Geometry check sheet. Reference: the model listing, model coordinates, mm. Face numbers are marked on the shaded views. A direction names the side the tool comes from. Coordinates: 2 decimals unless noted, no trailing zeros. Loops run counter-clockwise (first coordinate to the right, second up) from the corner with the lowest first, then second, coordinate; pieces in that order, holes last.
from build123d import *

# Parameters (mm, degrees)
BOSS_EXTRUDE1_DEPTH = 167.4876
FILLET1_R           = 4.7625
SHELL2_T            = -3.175
SKETCH2_R           = 25.4
CUT_EXTRUDE1_DEPTH  = 7.62


with BuildPart() as part:
    # Sketch1 → Boss-Extrude1 (new, symmetric)
    with BuildSketch(Plane(origin=(0, 0, 0), x_dir=(0, 0, -1), z_dir=(1, 0, 0))):
        Polygon((0, 0), (134.9502, 62.92831173), (134.9502, 113.72831173), (0, 113.72831173), align=None)
    extrude(amount=BOSS_EXTRUDE1_DEPTH, both=True)

    # Fillet1
    fillet1_edges = [part.edges().sort_by_distance(p)[0] for p in [
        (167.4876, 56.864155865, 0),
        (167.4876, 31.464155865, -67.4751),
        (167.4876, 88.32831173, -134.9502),
        (-167.4876, 31.464155865, -67.4751),
        (-167.4876, 56.864155865, 0),
        (-167.4876, 88.32831173, -134.9502),
        (0, 62.92831173, -134.9502),
        (0, 0, 0),
    ]]
    fillet(fillet1_edges, radius=FILLET1_R)

    # Shell2
    shell2_openings = [part.faces().sort_by_distance(p)[0] for p in [
        (0, 113.72831173, -67.4751),
    ]]
    offset(amount=SHELL2_T, openings=shell2_openings, kind=Kind.INTERSECTION)

    # Sketch2 → Cut-Extrude1 (cut)
    with BuildSketch(Plane(origin=(0, 0, 0), x_dir=(1, 0, 0), z_dir=(0, -0.9063077870366493, -0.422618261740701))):
        with Locations(Location((-124.5824, -79.05107084, 0), (0, 0, 270))):
            Circle(SKETCH2_R)
        with Locations(Location((-44.5824, -79.05107084, 0), (0, 0, 270))):
            Circle(SKETCH2_R)
        with Locations(Location((35.4176, -79.05107084, 0), (0, 0, 270))):
            Circle(SKETCH2_R)
        with Locations(Location((115.4176, -79.05107084, 0), (0, 0, 270))):
            Circle(SKETCH2_R)
    extrude(amount=-CUT_EXTRUDE1_DEPTH, mode=Mode.SUBTRACT)


solid = part.part
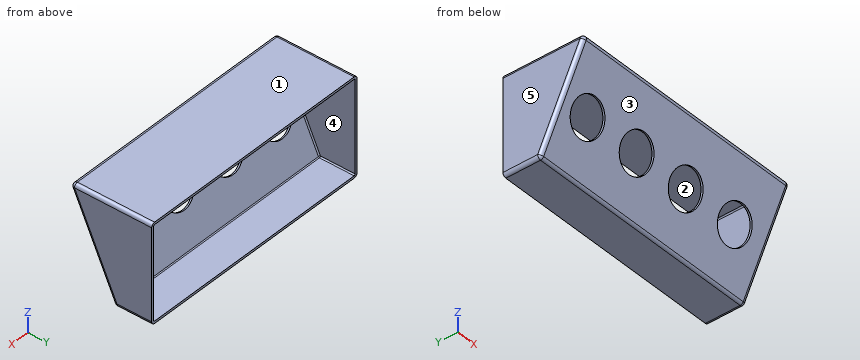
(1) Sectioned sample at A-A on y = 105. Record the cut outline in (x, z) (1 decimal).
Findings:
outline: (-167.5, -130.2) arc R4.8 ccw to (-162.7, -135) - (162.7, -135) arc R4.8 ccw to (167.5, -130.2) - (167.5, -4.8) arc R4.8 ccw to (162.7, 0) - (-162.7, 0) arc R4.8 ccw to (-167.5, -4.8) - close; hole (-164.3, -130.2) arc R1.6 ccw to (-162.7, -131.8) - (162.7, -131.8) arc R1.6 ccw to (164.3, -130.2) - (164.3, -4.8) arc R1.6 ccw to (162.7, -3.2) - (-162.7, -3.2) arc R1.6 ccw to (-164.3, -4.8) - close
(2) Sectioned sample at C-C on x = -92.5. Record the cut outline in (y, z) (1 decimal).
Findings:
outline: (3.2, -6.8) - (61.6, -132.2) arc R4.8 ccw to (66, -135) - (113.7, -135) - (113.7, -131.8) - (66, -131.8) arc R1.6 cw to (64.5, -130.9) - (6, -5.4) arc R1.6 cw to (7.5, -3.2) - (113.7, -3.2) - (113.7, 0) - (7.5, 0) arc R4.8 ccw to start
(3) Access from +Z, -Z, +X, -X, +Y, -Y to the whole of each face (thin tool, end or side, straight path). Record for the marked faces 1 and 2.
Findings:
face 1: +Z, +X, -X, +Y, -Y
face 2: +Y
(4) Draft check along Z on the marked faces 3, 4 and 5. Enter one of: +Z half, -Z half, draft (parallel to the pull), parting line (faces both ways), or undercut.
Findings:
face 3: -Z half
face 4: undercut
face 5: draft
(5) Gauge pin test, flat ends, axial feed: pin 1 Ø1.5 at (x, z) = (48.5, -87) entering from +Y; pin 2 Ø6 at (x, y) = (12.5, 28.5) entering from -Z; pin 3 Ø5 at (x, z) = (129.5, -26) entering from +Y; pin 4 Ø2 at (x, z) = (-65, -97) entering from -Y. Record the tip position at first contact, or that the pin passes through.
Findings:
pin 1: passes through
pin 2: stops at z = -66.29
pin 3: stops at y = 16.79
pin 4: stops at y = 44.77
(6) Sectioned sample at D-D on x = 129. Record the cut outline in (y, z) (1 decimal).
Findings:
outline: (3.2, -6.8) - (24.3, -52.2) - (27.2, -50.9) - (6, -5.4) arc R1.6 cw to (7.5, -3.2) - (113.7, -3.2) - (113.7, 0) - (7.5, 0) arc R4.8 ccw to start; (42.5, -91.1) - (61.6, -132.2) arc R4.8 ccw to (66, -135) - (113.7, -135) - (113.7, -131.8) - (66, -131.8) arc R1.6 cw to (64.5, -130.9) - (45.4, -89.8) - close
(7) Scan lines: L1, parallel to X at y = 73, z = -77; L2, parallel to Z at x = 138, y = 78 (3 decimals); L3, parallel to Z at x = 28, y = 14 (3 decimals). Record each from-to range of solid material in increasing order.
Findings:
L1: x = -167.49 to -164.31, 164.31 to 167.49
L2: z = -134.95 to -131.775, -3.175 to 0
L3: z = -30.023 to -22.51, -3.175 to 0
(8) Sectioned sample at B-B on x = 43. Record the cut outline in (y, z) (1 decimal), and give its area (3 significant figures).
Findings:
outline: (3.2, -6.8) - (23.2, -49.7) - (26, -48.3) - (6, -5.4) arc R1.6 cw to (7.5, -3.2) - (113.7, -3.2) - (113.7, 0) - (7.5, 0) arc R4.8 ccw to start; (43.7, -93.6) - (61.6, -132.2) arc R4.8 ccw to (66, -135) - (113.7, -135) - (113.7, -131.8) - (66, -131.8) arc R1.6 cw to (64.5, -130.9) - (46.5, -92.3) - close
area: 806 mm2
